Job drawing, mm, ordinate dimensions from the low corner. One solid piece. A direction names the side the tool comes from. Give positions to 0.01 mm unless a question says otherwise; leave off trailing zeros. Order: outer loops, then holes, each group sorted by start corner. A loop starts at its lowest first (then second) coordinate and runs counter-clockwise, first axis right, second up. Notation, with made-up numbers: M -15.5,38.5 L -1.5,38.5 A8 cw -1.5,53.5 Z; hole C 46.5,-31.75 d2. An arc over 180 degrees is marked long. Use CSV: the item, a comma, the result in double quotes. Start each with the question number.
Item 1: Which spindle directions (+Z, -Z, +X, -X, +Y, -Y) get a long thin tool onto all of the face, cutting with end or side? Do the marked faces 1 and 2. Say none if no direction does.
Item 2: Wall check: line 1 along Z through (x, y) = (72, 66); line 2 along Y through (x, z) = (6, 46.5); line 3 along Y through (x, z) = (11, 37). Give the ranges that are in metal, low to high.
Item 3: Pin check, flat tips, straight feed: P1, Ø1.5, axis at x = 54, y = 22.5, coming from the -Z side; P2, Ø6, axis at x = 44.5, y = 40, coming from the +Z side; P3, Ø12, axis at x = 19.5, z = 121.5, coming from the +Y side. Stop position of each tip, or through.
Item 4: Band-saw the part on B-B on x = 60.5. Write the cut outline in (y, z).
Item 5: Band-saw the part on A-A on y = 65. Write the cut outline in (x, z), plus the area to 3 significant figures.
Item 6: Band-saw the part on C-C on z = 41.5. Write the cut outline in (x, y), plus the area to 3 significant figures.
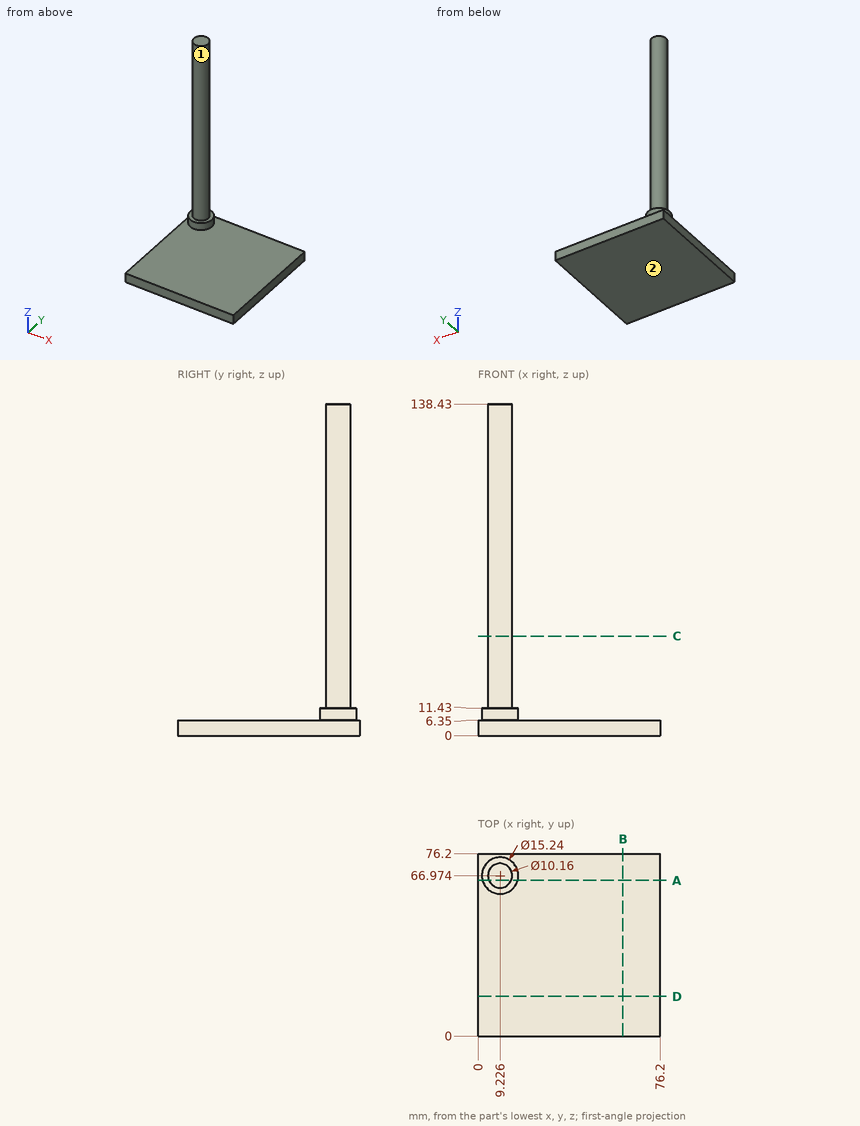
Model answer:
1,face 1,"+Z"
1,face 2,"-Z, +X, -X, +Y, -Y"
2,line 1,"z = 0 to 6.35"
2,line 2,"y = 63.05 to 70.9"
2,line 3,"y = 62.21 to 71.73"
3,P1,"stops at z = 0"
3,P2,"stops at z = 6.35"
3,P3,"stops at y = 69.72"
4,outline,"M 0,0 L 76.2,0 L 76.2,6.35 L 0,6.35 Z"
5,outline,"M 0,0 L 76.2,0 L 76.2,6.35 L 16.59,6.35 L 16.59,11.43 L 13.91,11.43 L 13.91,138.43 L 4.55,138.43 L 4.55,11.43 L 1.87,11.43 L 1.87,6.35 L 0,6.35 Z"
5,area,"1,750 mm^2"
6,outline,"C 9.23,66.97 d10.16"
6,area,"81.1 mm^2"
